Part model, mm, in its own coordinate system. A direction names the side the tool comes from. Coordinates: 2 decimals unless noted, no trailing zeros. Loops run counter-clockwise (first coordinate to the right, second up) from the corner with the lowest first, then second, coordinate; pieces in that order, holes last. Notation, with made-up numbers: M -24.5,43 L 33.5,43 A8 cw 33.5,49 Z; hole C -14.75,-28.75 d3. An arc over 180 degrees is marked long. Use a Markdown table: item, result. Add a question column.
1) Wall check: probe 1 along Y at (x, z) = (7.75, 17); probe 2 along Y at (x, z) = (5, 1); probe 3 along Z at (x, y) = (12, 16.5). Give the ranges that are in metal, low to high. Write a range as from..to.
2) Band-saw the part on D-D (x = 18.75). List the corners of the cut face in (y, z), plus the area to 4 significant figures.
3) Band-saw the part on B-B (y = 10). List the corners of the cut face in (x, z), plus the area to 3 significant figures.
4) Band-saw the part on A-A (x = 10). List the corners of the cut face in (y, z), plus the area to 3 significant figures.
5) Tool access for faces 1 (the flat face through (9.9, 2.5, 15.3)), 2 (the cylindrical face through (13, 8.5, 1.3)): list every direction of +Z, -Z, +X, -X, +Y, -Y with a clear straight run to the whole face (end or side of a thin tool).
6) Band-saw the part on C-C (z = 18). List the corners of the cut face in (x, y), plus the area to 3 significant figures.
7) Pull direction Z, two halves, no side cores. Call faces 3 (the cylindrical face through (14.77, 1.27, 8.5)), 4 (the flat face through (0, 9, 2)), 5 (the flat face through (10, 10, 0)), 6 (the cylindrical face through (14.77, 18.77, 8.5)): released by +Z, released by -Z, zero draft, split by the parting line, or undercut.
8) Pin check, flat tips, straight feed: pin 1 Ø7.5 at (x, y) = (11.5, 10.5) entering from +Z; pin 2 Ø5 at (x, z) = (11.5, 9.5) entering from -Y. Stop position of each tip, or through.
from build123d import *

# Parameters (mm, degrees)
SKETCH1_W           = 20
SKETCH1_H           = 20
BOSS_EXTRUDE1_DEPTH = 20
SKETCH2_W           = 20
SKETCH2_H           = 15
CUT_EXTRUDE1_DEPTH  = 17.5
SKETCH3_R           = 5
CUT_EXTRUDE2_DEPTH  = 21
SKETCH4_R           = 2.5
CUT_EXTRUDE3_DEPTH  = 3.5


with BuildPart() as part:
    # Sketch1 → Boss-Extrude1 (new body)
    with BuildSketch(Plane.XY):
        with Locations((10, 10)):
            Rectangle(SKETCH1_W, SKETCH1_H)
    extrude(amount=BOSS_EXTRUDE1_DEPTH)

    # Sketch2 → Cut-Extrude1 (cut)
    with BuildSketch(Plane.XY.offset(20)):
        with Locations((10, 10)):
            Rectangle(SKETCH2_W, SKETCH2_H)
    extrude(amount=-CUT_EXTRUDE1_DEPTH, mode=Mode.SUBTRACT)

    # Sketch3 → Cut-Extrude2 (cut, through all)
    with BuildSketch(Plane(origin=(0, 20, 0), x_dir=(1, 0, 0), z_dir=(0, 1, 0))):
        with Locations((10, -10)):
            Circle(SKETCH3_R)
    extrude(amount=-CUT_EXTRUDE2_DEPTH, mode=Mode.SUBTRACT)

    # Sketch4 → Cut-Extrude3 (cut, through all)
    with BuildSketch(Plane.XY.offset(2.5)):
        with Locations((15, 10)):
            Circle(SKETCH4_R)
        with Locations((5, 10)):
            Circle(SKETCH4_R)
    extrude(amount=-CUT_EXTRUDE3_DEPTH, mode=Mode.SUBTRACT)


solid = part.part
Entries:
| question | item | result |
|---|---|---|
| 1 | probe 1 | 0..2.5, 17.5..20 |
| 1 | probe 2 | 0..7.5, 12.5..20 |
| 1 | probe 3 | 0..2.5 |
| 2 | outline | M 0,0 L 20,0 L 20,20 L 17.5,20 L 17.5,2.5 L 2.5,2.5 L 2.5,20 L 0,20 Z |
| 2 | area | 137.5 mm2 |
| 3 | outline | M 0,0 L 2.5,0 L 2.5,2.5 L 0,2.5 Z; M 7.5,0 L 12.5,0 L 12.5,2.5 L 7.5,2.5 Z; M 17.5,0 L 20,0 L 20,2.5 L 17.5,2.5 Z |
| 3 | area | 25.0 mm2 |
| 4 | outline | M 0,0 L 20,0 L 20,5 L 17.5,5 L 17.5,2.5 L 2.5,2.5 L 2.5,5 L 0,5 Z; M 0,15 L 2.5,15 L 2.5,20 L 0,20 Z; M 17.5,15 L 20,15 L 20,20 L 17.5,20 Z |
| 4 | area | 87.5 mm2 |
| 5 | face 1 | +Z, +X, -X |
| 5 | face 2 | +Z, -Z |
| 6 | outline | M 0,0 L 20,0 L 20,2.5 L 0,2.5 Z; M 0,17.5 L 20,17.5 L 20,20 L 0,20 Z |
| 6 | area | 100 mm2 |
| 7 | face 3 | undercut |
| 7 | face 4 | zero draft |
| 7 | face 5 | released by -Z |
| 7 | face 6 | undercut |
| 8 | pin 1 | z = 2.5 |
| 8 | pin 2 | through |
